The model under review builds one solid part; all positions refer to its coordinate system, in mm. A direction names the side the tool comes from. Coordinates: 2 decimals unless noted, no trailing zeros. Order: outer loops, then holes, each group sorted by start corner. A loop starts at its lowest first (then second) coordinate and runs counter-clockwise, first axis right, second up.
```python
from build123d import *

# Parameters (mm, degrees)
F_3_5_3_5_DURCHMESSER_BOHRUNG1_D = 3.5
SKIZZE5_W                        = 0.5
SKIZZE5_H                        = 50
SCHNITT_LINEAR_AUSTRAGEN1_DEPTH  = 6


with BuildPart() as part:
    # Skizze1 → Rotation1 (revolve)
    with BuildSketch(Plane.XY):
        Polygon((-4, 0), (-4, 13.5), (-5.1, 13.5), (-5.1, 3.5), (-11, 3.5), (-11, 0), (-5.1, 0), (-5.1, -1.5), (-4, -1.5), align=None)
    revolve(axis=Axis((0, 0, 0), (0, 1, 0)))

    # Ø3.5 (3.5) Durchmesser Bohrung1 (through all)
    with Locations(Plane(origin=(0, 3.5, 0), x_dir=(1, 0, 0), z_dir=(0, 1, 0))):
        with Locations((5.656854249, 5.656854249), (-5.656854249, 5.656854249), (5.656854249, -5.656854249), (-5.656854249, -5.656854249)):
            Hole(F_3_5_3_5_DURCHMESSER_BOHRUNG1_D / 2)

    # Skizze5 → Schnitt-Linear austragen1 (cut, through all)
    with BuildSketch(Plane(origin=(0, 3.5, 0), x_dir=(1, 0, 0), z_dir=(0, 1, 0))):
        with Locations((-11, 0)):
            Rectangle(SKIZZE5_W, SKIZZE5_H)
    extrude(amount=-SCHNITT_LINEAR_AUSTRAGEN1_DEPTH, mode=Mode.SUBTRACT)


solid = part.part
```
(1) We need section A-A, the plane x = 0. Write out the cut boundary in (y, z).
A:
outline: (-1.5, -5.1) - (0, -5.1) - (0, -11) - (3.5, -11) - (3.5, -5.1) - (13.5, -5.1) - (13.5, -4) - (-1.5, -4) - close; (-1.5, 4) - (13.5, 4) - (13.5, 5.1) - (3.5, 5.1) - (3.5, 11) - (0, 11) - (0, 5.1) - (-1.5, 5.1) - close
(2) Machinability: for faces 4 (the face through (2, 3.5, -5)), 5 (the face through (-5, 0, 3)), 6 (the face through (11, 2, 0)), which of the approach directions +Z, -Z, +X, -X, +Y, -Y give a long, thin tool a straight path to every point of the face, cutting with its end or side? Answer none if there is none.
A:
face 4: +Y
face 5: -Y
face 6: +Y, -Y
(3) We need section D-D, the plane z = -9.25. Write out the cut boundary in (x, y), and give its area (3 significant figures).
A:
outline: (-5.95, 0) - (5.95, 0) - (5.95, 3.5) - (-5.95, 3.5) - close
area: 41.7 mm2
(4) For pin 1 Ø2 at (y, z) = (10.5, -5) entering from +X; pin 2 Ø3 at (x, z) = (-5.66, 5.66) entering from +Y; pin 3 Ø6 at (x, z) = (-8.5, -2) entering from -Y; pin 4 Ø5 at (x, y) = (7, 4) entering from -Z, all flat-tipped, find the tip position at first contact; note any pin that passes through.
A:
pin 1: stops at x = 3.16
pin 2: passes through
pin 3: stops at y = 0
pin 4: stops at z = -10.01
(5) We need section B-B, the plane y = 5.5. Write out the cut boundary in (x, z), and give its area (3 significant figures).
A:
outline: circle Ø10.2 at (0, 0); hole circle Ø8 at (0, 0)
area: 31.4 mm2
(6) Wall thickness on probe 1 along Z at (x, y) = (0, 3); probe 2 along X at (y, z) = (1, -6.25); probe 3 along Z at (x, y) = (5, 0.25): over which ranges is each line inside the solid? List them lowest first.
A:
probe 1: z = -11 to -4, 4 to 11
probe 2: x = -9.05 to -7.3, -4.01 to 4.01, 7.3 to 9.05
probe 3: z = -9.8 to -7.28, -4.03 to 4.03, 7.28 to 9.8
(7) We need section C-C, the plane y = 1. Write out the cut boundary in (x, z).
A:
outline: (-10.75, -2.33) arc R11 ccw (long way) to (-10.75, 2.33) - close; hole circle Ø3.5 at (-5.66, -5.66); hole circle Ø3.5 at (-5.66, 5.66); hole circle Ø8 at (0, 0); hole circle Ø3.5 at (5.66, -5.66); hole circle Ø3.5 at (5.66, 5.66)
(8) Draft analysis for pull direction X (two halves, no side actions). For faces 1 (the face through (3, -1.5, -3)), 2 (the face through (0.867, 6.105, -3.905)), 3 (the face through (-2.4, -0.8, -4.5)), state which applies: released by +X, released by -X, zero draft, split by the parting line, or undercut.
A:
face 1: zero draft
face 2: undercut
face 3: split by the parting line
